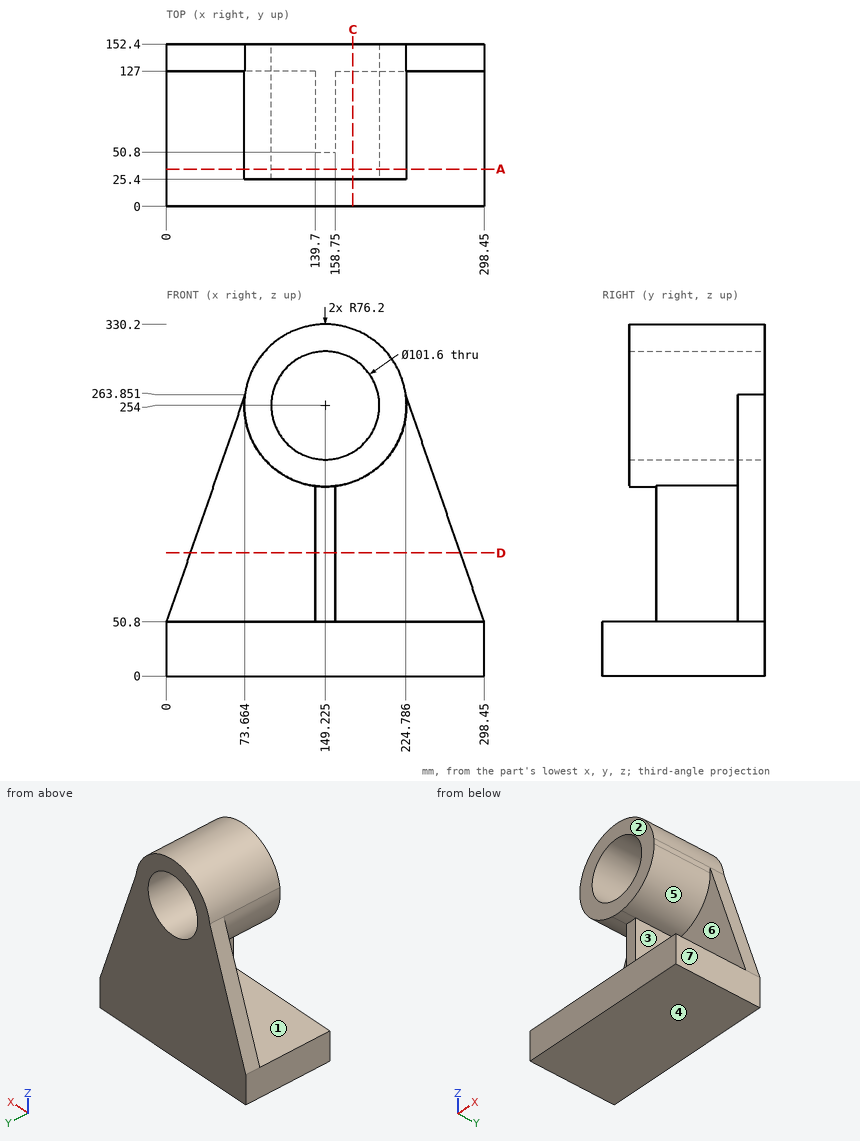
Source: three-view drawing plus pictorial views. Frame: mm from the lowest corner of the part. A direction names the side the tool comes from. Give positions to 0.01 mm unless a question says otherwise; leave off trailing zeros. Write each loop counter-clockwise with the first axis right and the second up, starting at its lowest first coordinate (ties: lowest second). Pieces come first, ordered by that corner, then holes.
(1) Mould query, pull axis Z, two halves, no side actions, for the marked faces 4, 5, 6 and 7. Classes: released by +Z, released by -Z, zero draft, split by the parting line, or undercut.
(2) Cut plane A-A, the plane y = 35. Give the number of separate pieces and of enclosed holes in the cut face, then the cut area to 3 significant figures.
(3) First-contact query: P1, Ø4, axis at x = 98.5, z = 294.5, coming from the -Y side; P2, Ø3, axis at x = 265, z = 155, coming from the -Y side; P3, Ø2, axis at x = 149, y = 39, coming from the +Z side; P4, Ø1, axis at y = 121, z = 209.5, coming from the +X side. Flat tips, straight axial feed; report the tip coordinate or a pass-through.
(4) Ray query, line 1 (Z direction, x = 150.5, y = 50); line 2 (Z direction, x = 186, y = 111.5) (1 decimal); line 3 (X direction, y = 74.5, z = 58.5). Return the intervals inside material, ascending.
(5) Cut plane C-C, the plane x = 175. Return loops of the section in (y, z) (1 decimal), then the cut area to 3 significant figures.
(6) Cut plane D-D, the plane z = 115.5. Return loops of the section in (x, y), then the cut area to 3 significant figures.
(7) Access query for the marked faces 1, 2 and 3. Directions: +Z, -Z, +X, -X, +Y, -Y. A direction counts if a zero-diameter tool reaches every point of the face in a straight line with its end or side. Return the directions, or none.
Values follow:
1. face 4: released by -Z
1. face 5: undercut
1. face 6: undercut
1. face 7: zero draft
2. separate pieces: 2
2. enclosed holes: 1
2. area: 25,300 mm2
3. P1: stops at y = 25.4
3. P2: passes through
3. P3: stops at z = 330.2
3. P4: stops at x = 211.44
4. line 1: z = 0 to 50.8, 177.81 to 203.22, 304.78 to 330.19
4. line 2: z = 0 to 50.8, 187.3 to 219, 289 to 320.7
4. line 3: x = 139.7 to 158.75
5. outline: (0, 0) - (152.4, 0) - (152.4, 210.2) - (25.4, 210.2) - (25.4, 182.3) - (127, 182.3) - (127, 50.8) - (0, 50.8) - close; (25.4, 297.8) - (152.4, 297.8) - (152.4, 325.7) - (25.4, 325.7) - close
5. area: 18,200 mm2
6. outline: (22.37, 127) - (139.7, 127) - (139.7, 50.8) - (158.75, 50.8) - (158.75, 127) - (276.08, 127) - (276.08, 152.4) - (22.37, 152.4) - close
6. area: 7,900 mm2
7. face 1: -Y
7. face 2: +Z, +X, -X, -Y
7. face 3: +X, -Y
